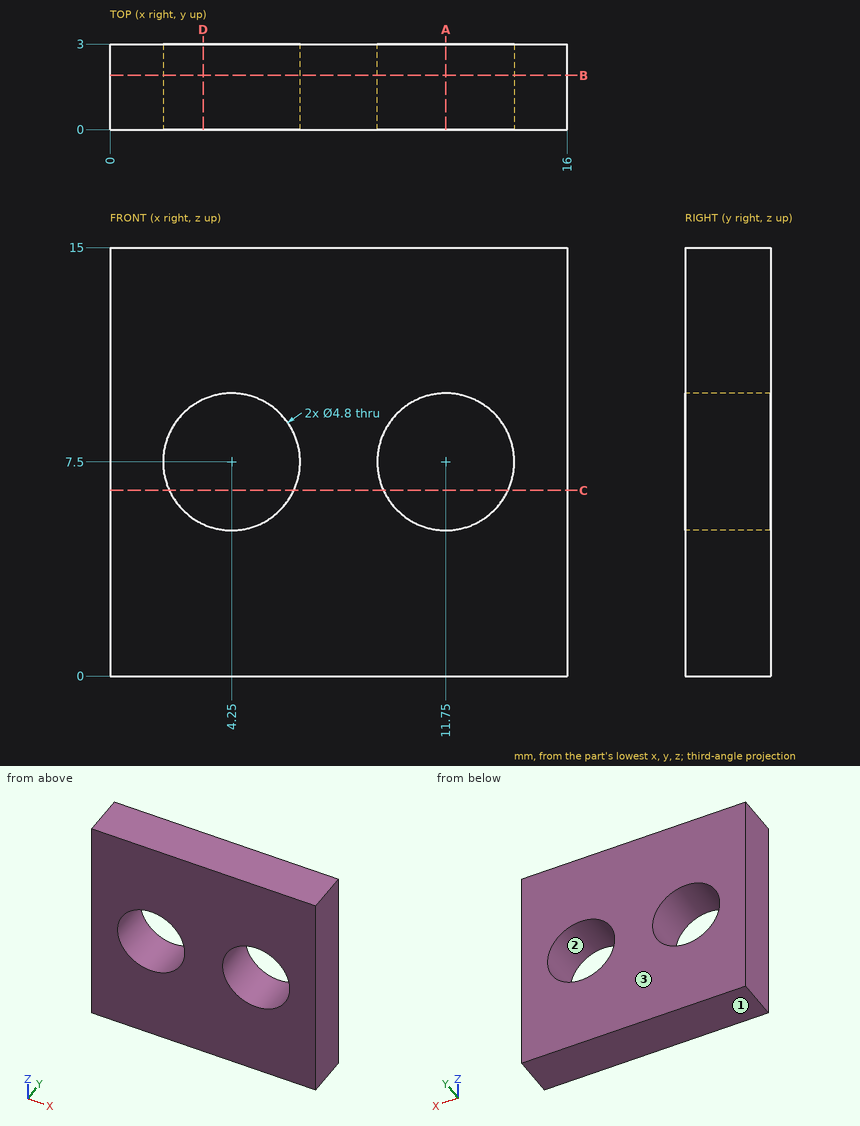
Verification items for this drawing (mm, ordinates from the low corner). Give positions to 0.01 mm unless a question says otherwise; leave off trailing zeros. Write each loop counter-clockwise with the first axis right and the second up, starting at its lowest first coordinate (ties: lowest second). Pieces come first, ordered by that corner, then holes. Notation, with made-up numbers: (44.5, 84.25) -> (90.5, 84.25) arc R24 ccw to (90.5, 116.25) -> close; hole circle Ø8 at (78.5, -10). An arc over 180 degrees is marked (long way). Use CSV: the item, a comma, the result in double quotes.
(1) Material ranges on L1, parallel to Z at x = 11.75, y = 0.2; L2, parallel to X at y = 1.7, z = 8; L3, parallel to X at y = 1.3, z = 5.5, recorded low to high.
Derived:
L1,"z = 0 to 5.1, 9.9 to 15"
L2,"x = 0 to 1.9, 6.6 to 9.4, 14.1 to 16"
L3,"x = 0 to 2.92, 5.58 to 10.42, 13.08 to 16"
(2) Sectioned sample at D-D (x = 3.25). Record the cut outline in (y, z).
Derived:
outline,"(0, 0) -> (3, 0) -> (3, 5.32) -> (0, 5.32) -> close; (0, 9.68) -> (3, 9.68) -> (3, 15) -> (0, 15) -> close"
(3) Sectioned sample at A-A (x = 11.75). Record the cut outline in (y, z), plus the area to 3 significant figures.
Derived:
outline,"(0, 0) -> (3, 0) -> (3, 5.1) -> (0, 5.1) -> close; (0, 9.9) -> (3, 9.9) -> (3, 15) -> (0, 15) -> close"
area,"30.6 mm^2"
(4) Release check for a two-part mould opening along Z. For the marked faces 1, 2 and 3 record: +Z half, -Z half, draft (parallel to the pull), parting line (faces both ways), or undercut.
Derived:
face 1,"-Z half"
face 2,"undercut"
face 3,"draft"
(5) Sectioned sample at C-C (z = 6.5). Record the cut outline in (x, y).
Derived:
outline,"(0, 0) -> (2.07, 0) -> (2.07, 3) -> (0, 3) -> close; (6.43, 0) -> (9.57, 0) -> (9.57, 3) -> (6.43, 3) -> close; (13.93, 0) -> (16, 0) -> (16, 3) -> (13.93, 3) -> close"
(6) Sectioned sample at B-B (y = 1.9). Record the cut outline in (x, z), plus the area to 3 significant figures.
Derived:
outline,"(0, 0) -> (16, 0) -> (16, 15) -> (0, 15) -> close; hole circle Ø4.8 at (4.25, 7.5); hole circle Ø4.8 at (11.75, 7.5)"
area,"204 mm^2"
